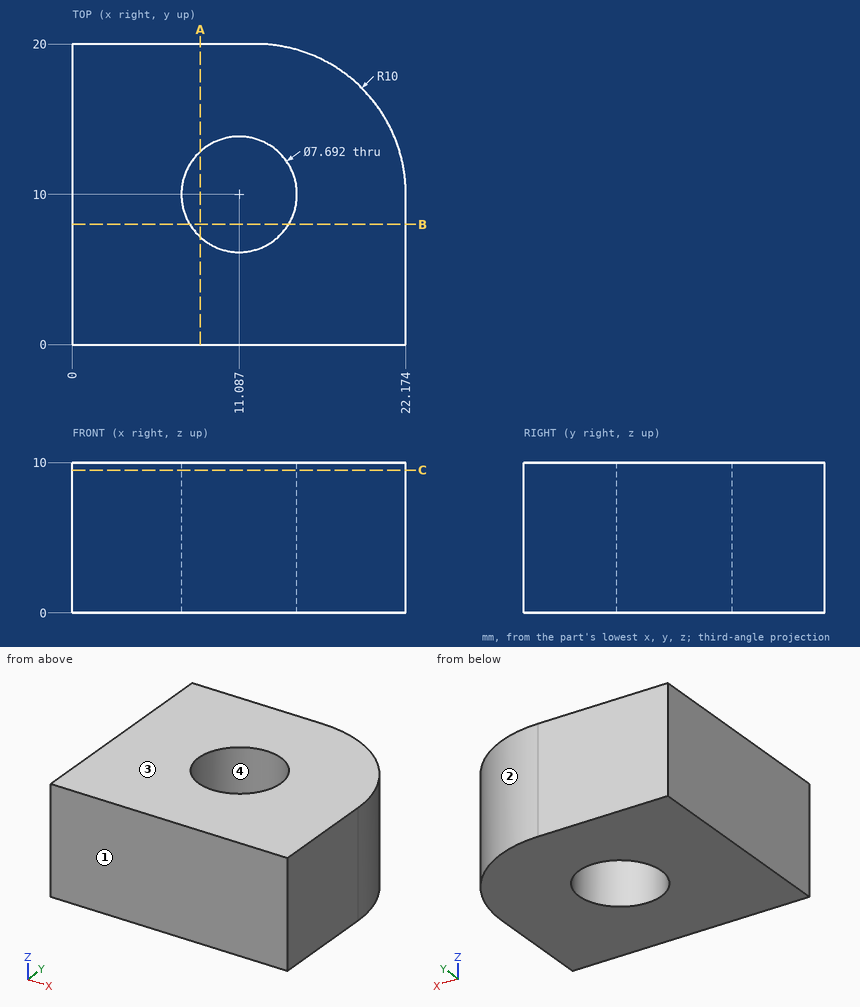
Here's the drawing with two shaded views (mm, measured from the low corner). I have some questions. Give positions to 0.01 mm unless a question says otherwise; leave off trailing zeros. Loops run counter-clockwise (first coordinate to the right, second up) from the corner with the lowest first, then second, coordinate; pieces in that order, holes last. Notation, with made-up numbers: (19, -2.75) -> (77, -2.75) arc R20 ccw to (77, 30.25) -> close; hole circle Ø11 at (-13.75, 87.5). An arc over 180 degrees is marked (long way). One line per item, written item: value.
Q1. Suppose I cut it at B-B on y = 8. Please give me the cut outline in (x, z).
Answers follow:
outline: (0, 0) -> (7.8, 0) -> (7.8, 10) -> (0, 10) -> close; (14.37, 0) -> (22.17, 0) -> (22.17, 10) -> (14.37, 10) -> close
Q2. I'm going to push flat-ended pins straight in: pin 1 Ø1.5 at (x, z) = (14.5, 6) entering from +Y (3 decimals); pin 2 Ø2 at (y, z) = (17.5, 8.5) entering from +X. Where does each tip first touch, or does it pass through?
Answers follow:
pin 1: y = 19.875
pin 2: x = 19.77
Q3. If I drill on line 1 along X through (y, z) = (9.25, 1.75) (1 decimal); line 2 along Y through (x, z) = (14, 2.5); line 3 along Y through (x, z) = (8.75, 6) (1 decimal), over which ranges is the centre line in solid material (lowest first)?
Answers follow:
line 1: 0 to 7.3, 14.9 to 22.2
line 2: 0 to 7.49, 12.51 to 19.83
line 3: 0 to 6.9, 13.1 to 20
Q4. Suppose I cut it at C-C on z = 9.5. Please give me the cut outline in (x, y), then the cut area to 3 significant figures.
Answers follow:
outline: (0, 0) -> (22.17, 0) -> (22.17, 10) arc R10 ccw to (12.17, 20) -> (0, 20) -> close; hole circle Ø7.69 at (11.09, 10)
area: 376 mm^2
Q5. Suppose I cut it at A-A on x = 8.5. Please give me the cut outline in (y, z), then the cut area to 3 significant figures.
Answers follow:
outline: (0, 0) -> (7.15, 0) -> (7.15, 10) -> (0, 10) -> close; (12.85, 0) -> (20, 0) -> (20, 10) -> (12.85, 10) -> close
area: 143 mm^2
Q6. We'd pull the mould along Y, two halves only. Please class the marked faces 1, 2, 3 and 4: pulls with the +Y half, pulls with the -Y half, needs draft (parallel to the pull), parting line crosses it, or undercut.
Answers follow:
face 1: pulls with the -Y half
face 2: pulls with the +Y half
face 3: needs draft
face 4: undercut
